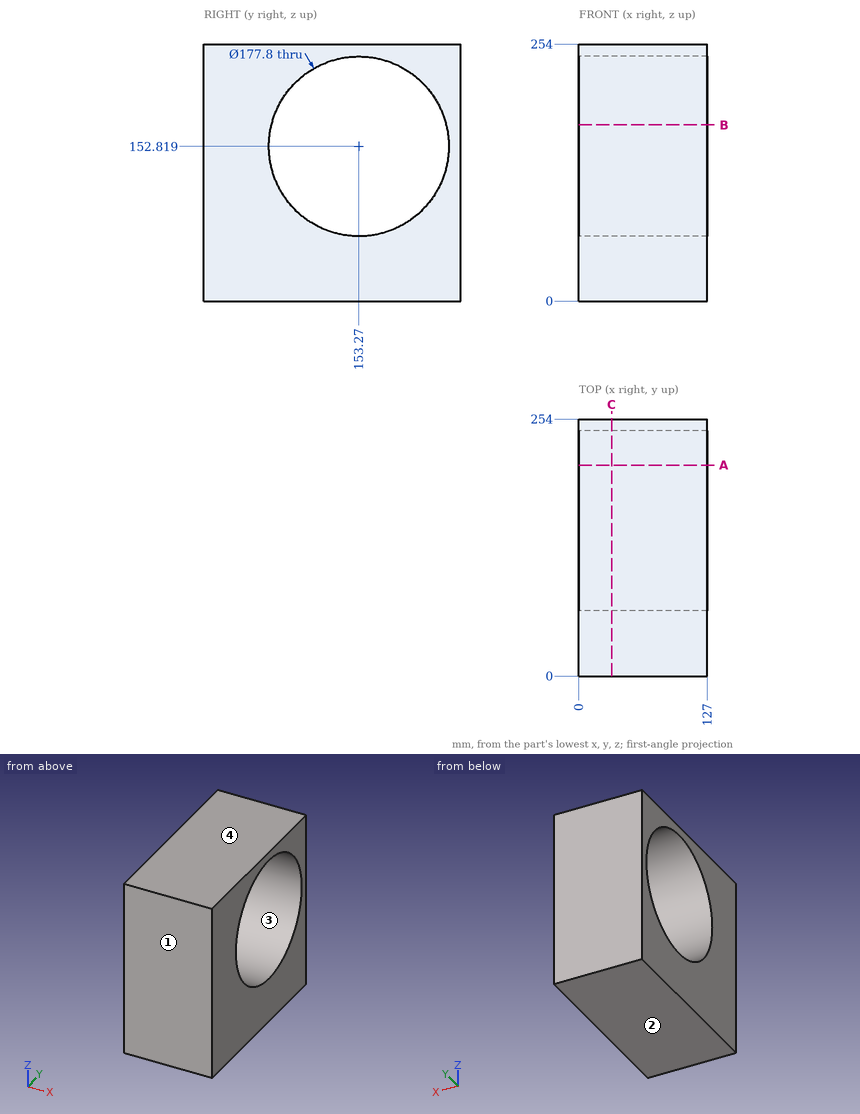
The drawing under review shows one solid part. Ordinate dimensions are in mm from its lowest x, y, z. Round coordinates to 2 decimals unless told otherwise and drop trailing zeros. Loops run counter-clockwise (first coordinate to the right, second up) from the corner with the lowest first, then second, coordinate; pieces in that order, holes last. Notation, with made-up numbers: (76.5, 74) - (123.5, 74) arc R25 cw to (123.5, 103) - close; hole circle Ø6 at (63, 75). An arc over 180 degrees is marked (long way). Use a Markdown table: item, result. Add a question column.
Q1. Add section A-A (y = 208.5). State the section outline as (x, z) points.
Q2. Add section C-C (x = 32.5). State the section outline as (y, z) points.
Q3. The part is to be moulded in two halves that separate along Z. For the marked faces 1, 2, 3 and 4, say which applies: pulls with the +Z half, pulls with the -Z half, needs draft (parallel to the pull), parting line crosses it, or undercut.
Q4. Add section B-B (z = 174). State the section outline as (x, y) points, plus the area to 3 significant figures.
Q5. For probe 1 along Y at (x, z) = (72.5, 108) (1 decimal); probe 2 along Z at (x, y) = (71, 164.5); probe 3 along Y at (x, z) = (76, 157), list the stretches that pass through material, from the lowest coordinate up.
Worked answers:
| question | item | result |
|---|---|---|
| 1 | outline | (0, 0) - (127, 0) - (127, 83.16) - (0, 83.16) - close; (0, 222.48) - (127, 222.48) - (127, 254) - (0, 254) - close |
| 2 | outline | (0, 0) - (254, 0) - (254, 254) - (0, 254) - close; hole circle Ø177.8 at (153.27, 152.82) |
| 3 | face 1 | needs draft |
| 3 | face 2 | pulls with the -Z half |
| 3 | face 3 | undercut |
| 3 | face 4 | pulls with the +Z half |
| 4 | outline | (0, 0) - (127, 0) - (127, 66.93) - (0, 66.93) - close; (0, 239.61) - (127, 239.61) - (127, 254) - (0, 254) - close |
| 4 | area | 10,300 mm² |
| 5 | probe 1 | 0 to 76.5, 230 to 254 |
| 5 | probe 2 | 0 to 64.63, 241.01 to 254 |
| 5 | probe 3 | 0 to 64.47, 242.07 to 254 |
